```python
from build123d import *

# Parameters (mm, degrees)
F0_R     = 1.5
F1_DEPTH = 4.5
F2_R     = 3


with BuildPart() as f1:
    # F0 (on Top) → F1 (new body)
    with BuildSketch(Plane.XY):
        with BuildLine():
            Line((22.091176, 20.297059), (-20.208824, 20.297059))
            Line((-20.208824, 20.297059), (-20.208824, -22.002941))
            Line((-20.208824, -22.002941), (-10.308824, -22.002941))
            Line((-10.308824, -22.002941), (-10.308824, -1.102941))
            ThreePointArc((-10.308824, -1.102941), (0.691176, 9.897059), (11.691176, -1.102941))
            Line((11.691176, -1.102941), (11.691176, -22.002941))
            Line((11.691176, -22.002941), (22.091176, -22.002941))
            Line((22.091176, -22.002941), (22.091176, 20.297059))
        make_face()
        with Locations((-14.308824, -16.102941)):
            Circle(F0_R, mode=Mode.SUBTRACT)
        with Locations((16.191176, -16.102941)):
            Circle(F0_R, mode=Mode.SUBTRACT)
        with Locations((-14.308824, 14.397059)):
            Circle(F0_R, mode=Mode.SUBTRACT)
        with Locations((16.191176, 14.397059)):
            Circle(F0_R, mode=Mode.SUBTRACT)
    extrude(amount=F1_DEPTH)

    # F2
    f2_edges = [f1.edges().sort_by_distance(p)[0] for p in [
        (11.691176, -22.002941, 2.25),
        (-10.308824, -22.002941, 2.25),
        (-20.208824, -22.002941, 2.25),
        (-20.208824, 20.297059, 2.25),
    ]]
    fillet(f2_edges, radius=F2_R)


solid = f1.part
```
For this review, take the finished solid that the model builds, in its own axes (mm). A direction names the side the tool comes from. Coordinates: 2 decimals unless noted, no trailing zeros. Order: outer loops, then holes, each group sorted by start corner. A loop starts at its lowest first (then second) coordinate and runs counter-clockwise, first axis right, second up. Notation, with made-up numbers: (40.25, 84) -> (72.25, 84) arc R11 cw to (72.25, 102) -> close; hole circle Ø1 at (-21, 53). An arc over 180 degrees is marked (long way). Use CSV: the item, a comma, the result in double quotes. Start each with the question number.
Item 1: Draft analysis for pull direction X (two halves, no side actions). For faces 3 (the face through (11.691, -10, 2)), 4 (the face through (-19.353, -21.101, 2.282)), 5 (the face through (1, 14, 0)), 6 (the face through (14.693, -16.037, 2.218)), state which applies: pulls with the +X half, pulls with the -X half, needs draft (parallel to the pull), parting line crosses it, or undercut.
Item 2: Wall thickness on probe 1 along X at (y, z) = (-5.5, 2.75); probe 2 along X at (y, z) = (-17, 1.4); probe 3 along Y at (x, z) = (0.5, 1.7): over which ranges is each line inside the solid? List them lowest first.
Item 3: We need section B-B, the plane y = -17. Give the boundary of the cut face in (x, z).
Item 4: We need section D-D, the plane y = 7.5. Give the boundary of the cut face in (x, z).
Item 5: We need section C-C, the plane z = 2.25. Give the boundary of the cut face in (x, y).
Item 6: Insertion check: pin 1 (1 mm diameter, centred on x = -11.5, z = 2, fed in from -Y). The pin has a flat end and moves straight along its axis. Give the tip position at first contact, or say it passes through.
Item 7: We need section A-A, the plane y = -8. Give the boundary of the cut face in (x, z).
Item 8: For faces 1 (the face through (-10.309, -10, 2)), 2 (the face through (-20.209, -1, 2)), list the 3-axis set-ups (+Z, -Z, +X, -X, +Y, -Y) from which the entire face can be reached by the end or side of a thin tool; tool diameter is ignored.
Derived:
1,face 3,"undercut"
1,face 4,"pulls with the -X half"
1,face 5,"needs draft"
1,face 6,"undercut"
2,probe 1,"x = -20.21 to -10.31, 11.69 to 22.09"
2,probe 2,"x = -20.21 to -15.51, -13.11 to -10.31, 11.69 to 14.99, 17.39 to 22.09"
2,probe 3,"y = 9.9 to 20.3"
3,outline,"(-20.21, 0) -> (-15.51, 0) -> (-15.51, 4.5) -> (-20.21, 4.5) -> close; (-13.11, 0) -> (-10.31, 0) -> (-10.31, 4.5) -> (-13.11, 4.5) -> close; (11.69, 0) -> (14.99, 0) -> (14.99, 4.5) -> (11.69, 4.5) -> close; (17.39, 0) -> (22.09, 0) -> (22.09, 4.5) -> (17.39, 4.5) -> close"
4,outline,"(-20.21, 0) -> (-6.16, 0) -> (-6.16, 4.5) -> (-20.21, 4.5) -> close; (7.55, 0) -> (22.09, 0) -> (22.09, 4.5) -> (7.55, 4.5) -> close"
5,outline,"(-20.21, -19) arc R3 ccw to (-17.21, -22) -> (-13.31, -22) arc R3 ccw to (-10.31, -19) -> (-10.31, -1.1) arc R11 cw to (11.69, -1.1) -> (11.69, -19) arc R3 ccw to (14.69, -22) -> (22.09, -22) -> (22.09, 20.3) -> (-17.21, 20.3) arc R3 ccw to (-20.21, 17.3) -> close; hole circle Ø3 at (-14.31, -16.1); hole circle Ø3 at (-14.31, 14.4); hole circle Ø3 at (16.19, -16.1); hole circle Ø3 at (16.19, 14.4)"
6,pin 1,"stops at y = -21.7"
7,outline,"(-20.21, 0) -> (-10.31, 0) -> (-10.31, 4.5) -> (-20.21, 4.5) -> close; (11.69, 0) -> (22.09, 0) -> (22.09, 4.5) -> (11.69, 4.5) -> close"
8,face 1,"+Z, -Z, -Y"
8,face 2,"+Z, -Z, -X, +Y, -Y"
